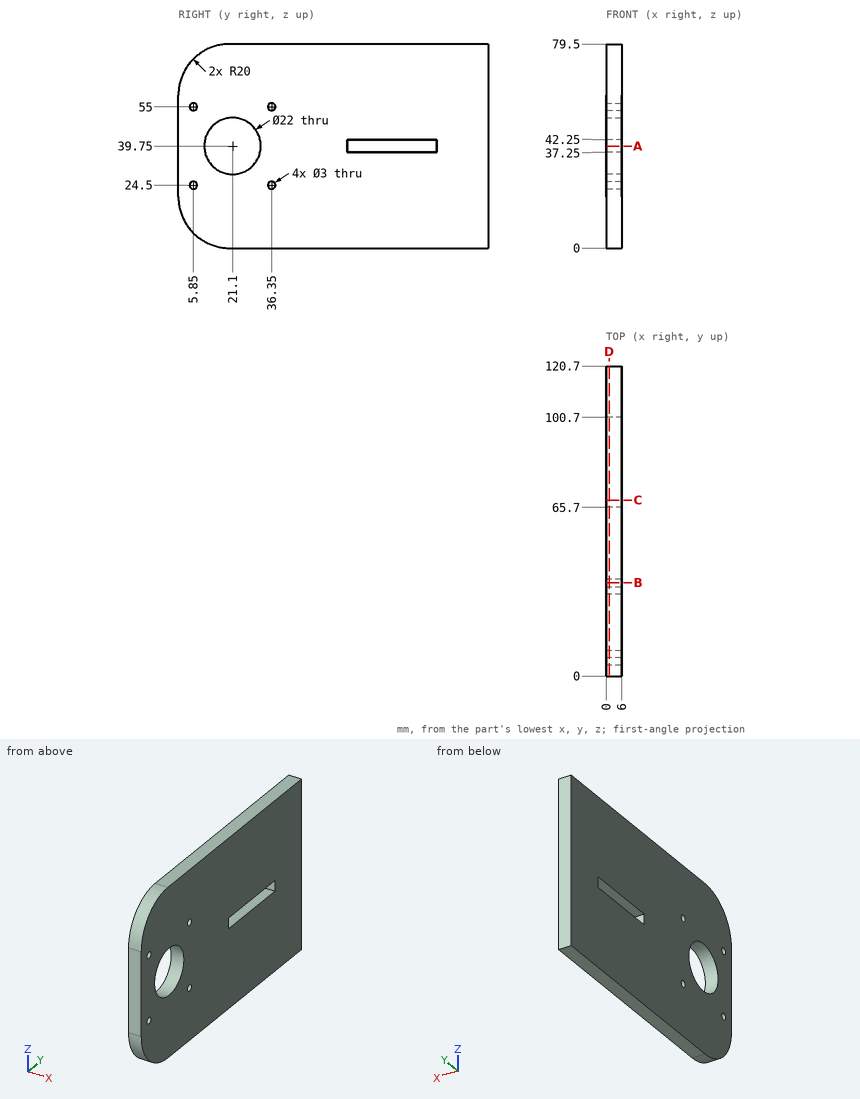
Verification items for this drawing (mm, ordinates from the low corner). Coordinates: 2 decimals unless noted, no trailing zeros. Write each loop counter-clockwise with the first axis right and the second up, starting at its lowest first coordinate (ties: lowest second). Pieces come first, ordered by that corner, then holes. Notation, with made-up numbers: M -25.75,77.5 L 27.25,77.5 A17 cw 27.25,91.5 Z; hole C -34.5,-6.5 d2. An arc over 180 degrees is marked long. Use one line per item in the form item = value. Start each with the question number.
1) Section check A-A on z = 39.75. Enter the section's corners in (x, y), and give its area (3 significant figures).
2) Section check D-D on x = 1.15. Enter the section's corners in (y, z), and give its area (3 significant figures).
3) Section check C-C on y = 68.5. Enter the section's corners in (x, z).
4) Section check B-B on y = 36.35. Enter the section's corners in (x, z).
5) Thickness scan on probe 1 along Y at (x, z) = (4.1, 55); probe 2 along Z at (x, y) = (4.25, 80); probe 3 along Z at (x, y) = (5.65, 23). Record the ranges inside material, lowest first. Write a range as from..to.
Responses:
q1.outline = M 0,0 L 6,0 L 6,10.1 L 0,10.1 Z; M 0,32.1 L 6,32.1 L 6,65.7 L 0,65.7 Z; M 0,100.7 L 6,100.7 L 6,120.7 L 0,120.7 Z
q1.area = 382 mm2
q2.outline = M 0,20 A20 ccw 20,0 L 120.7,0 L 120.7,79.5 L 20,79.5 A20 ccw 0,59.5 Z; hole C 5.85,24.5 d3; hole C 5.85,55 d3; hole C 21.1,39.75 d22; hole C 36.35,24.5 d3; hole C 36.35,55 d3; hole M 65.7,37.25 L 100.7,37.25 L 100.7,42.25 L 65.7,42.25 Z
q2.area = 8,840 mm2
q3.outline = M 0,0 L 6,0 L 6,37.25 L 0,37.25 Z; M 0,42.25 L 6,42.25 L 6,79.5 L 0,79.5 Z
q4.outline = M 0,0 L 6,0 L 6,23 L 0,23 Z; M 0,26 L 6,26 L 6,53.5 L 0,53.5 Z; M 0,56.5 L 6,56.5 L 6,79.5 L 0,79.5 Z
q5.probe_1 = 0..4.35, 7.35..34.85, 37.85..120.7
q5.probe_2 = 0..37.25, 42.25..79.5
q5.probe_3 = 0..28.92, 50.58..79.5
